Check sheet for the modelled part. Datum: model origin and axes. Units: mm. A direction names the side the tool comes from. Coordinates: 2 decimals unless noted, no trailing zeros. Loops run counter-clockwise (first coordinate to the right, second up) from the corner with the lowest first, then second, coordinate; pieces in that order, holes last. Notation, with made-up numbers: (38, 17) -> (84, 17) arc R20 ccw to (84, 46) -> close; hole circle Ø9 at (16, 55.5). An arc over 180 degrees is marked (long way). Use CSV: the item, a comma, the result in double quotes.
```python
from build123d import *

# Parameters (mm, degrees)
BOSS_EXTRUDE1_DEPTH = 6.35


with BuildPart() as part:
    # Sketch1 → Boss-Extrude1 (new body)
    with BuildSketch(Plane.XY):
        Polygon((0, 8.89), (8.89, 0), (5.926666667, 0), (5.926666667, -6.35), (2.963333333, -6.35), (2.963333333, 0), (0, 0), (0, 2.963333333), (-6.35, 2.963333333), (-6.35, 5.926666667), (0, 5.926666667), align=None)
    extrude(amount=BOSS_EXTRUDE1_DEPTH)


solid = part.part
```
1) Cross-section at C-C on x = 2. Record the boundary of the cut face in (y, z), and give its area (3 significant figures).
Answer below:
outline,"(0, 0) -> (6.89, 0) -> (6.89, 6.35) -> (0, 6.35) -> close"
area,"43.8 mm²"
2) Cross-section at B-B on y = 2.5. Record the boundary of the cut face in (x, z), and give its area (3 significant figures).
Answer below:
outline,"(0, 0) -> (6.39, 0) -> (6.39, 6.35) -> (0, 6.35) -> close"
area,"40.6 mm²"
3) Thickness scan on line 1 along X through (y, z) = (-2.5, 5.5); line 2 along X through (y, z) = (3.25, 3.5). Record the ranges inside material, lowest first. Write a range as from..to.
Answer below:
line 1,"x = 2.96..5.93"
line 2,"x = -6.35..5.64"
4) Access from +Z, -Z, +X, -X, +Y, -Y to the whole of each face (thin tool, end or side, straight path). Record for faces 1 (the flat face through (4, -6.35, 3)), 2 (the flat face through (-3, 5.927, 3)), 3 (the flat face through (7, 0, 3)), 4 (the flat face through (0, 1, 3)), 5 (the flat face through (2, 2, 0)).
Answer below:
face 1,"+Z, -Z, +X, -X, -Y"
face 2,"+Z, -Z, -X, +Y"
face 3,"+Z, -Z, +X, -Y"
face 4,"+Z, -Z, -X, -Y"
face 5,"-Z, +X, -X, +Y, -Y"
5) Go/stop test with flat-tipped pins: pin 1 Ø3 at (y, z) = (-3, 2.5) entering from +X; pin 2 Ø0.9 at (y, z) = (7, 3.5) entering from -X; pin 3 Ø5 at (x, y) = (0.5, -2.5) entering from +Z; pin 4 Ø1.5 at (x, z) = (1, 4.5) entering from -Y. Record where each tip stops, or that it passes through.
Answer below:
pin 1,"stops at x = 5.93"
pin 2,"stops at x = 0"
pin 3,"stops at z = 6.35"
pin 4,"stops at y = 0"
6) Cross-section at A-A on z = 4. Record the boundary of the cut face in (x, y).
Answer below:
outline,"(-6.35, 2.96) -> (0, 2.96) -> (0, 0) -> (2.96, 0) -> (2.96, -6.35) -> (5.93, -6.35) -> (5.93, 0) -> (8.89, 0) -> (0, 8.89) -> (0, 5.93) -> (-6.35, 5.93) -> close"
